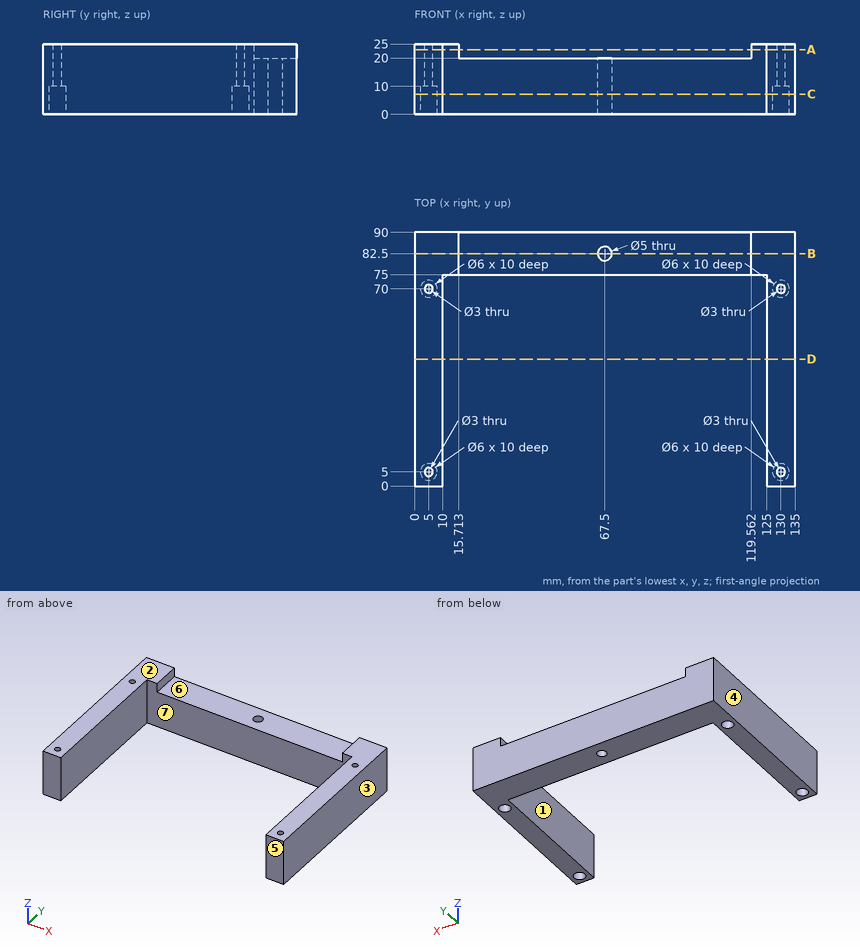
Could you check a few things on this drawing? It's one solid part, dimensions in mm from its lowest x, y, z. A direction names the side the tool comes from. Give positions to 0.01 mm unless a question says otherwise; leave off trailing zeros. Loops run counter-clockwise (first coordinate to the right, second up) from the corner with the lowest first, then second, coordinate; pieces in that order, holes last. Notation, with made-up numbers: (23, -2) -> (49, -2) arc R27 ccw to (49, 18) -> close; hole circle Ø3 at (74, 71). An arc over 180 degrees is marked (long way). Answer as CSV lines item,"result". Start each with the question number.
(1) If we section it at A-A on z = 23: Write out the boundary of the cut face in (x, y).
(2) If we section it at C-C on z = 7.25: Write out the boundary of the cut face in (x, y), then the cut area to 3 significant figures.
(3) I'm going to push flat-ended pins straight in: pin 1 Ø2 at (x, z) = (57, 17.5) entering from -Y; pin 2 Ø4.5 at (x, y) = (75, 84) entering from +Z; pin 3 Ø3 at (x, y) = (5.5, 5.5) entering from -Z. Where does each tip first touch, or does it pass through?
(4) We'd pull the mould along X, two halves only. Please class the marked faces 1, 2, 3 and 4: released by +X, released by -X, zero draft, split by the parting line, or undercut.
(5) If we section it at B-B on y = 82.5: Write out the boundary of the cut face in (x, z).
(6) I need wall thicknesses on probe 1 along X at (y, z) = (70, 15.75); probe 2 along X at (y, z) = (56, 10); probe 3 along Y at (x, z) = (129.5, 20.25) (1 decimal). Which ranges of each line are inside material? Lowest first, please.
(7) If we section it at D-D on y = 45: Write out the boundary of the cut face in (x, z), then the cut area to 3 significant figures.
(8) Which directions (+Z, -Z, +X, -X, +Y, -Y) give clear straight access to the entire face, cutting with the end or side of a thin tool? Please do the marked faces 5, 6 and 7.
Computed:
1,outline,"(0, 0) -> (10, 0) -> (10, 75) -> (15.71, 75) -> (15.71, 90) -> (0, 90) -> close; (119.56, 75) -> (125, 75) -> (125, 0) -> (135, 0) -> (135, 90) -> (119.56, 90) -> close; hole circle Ø3 at (5, 5); hole circle Ø3 at (5, 70); hole circle Ø3 at (130, 5); hole circle Ø3 at (130, 70)"
2,outline,"(0, 0) -> (10, 0) -> (10, 75) -> (125, 75) -> (125, 0) -> (135, 0) -> (135, 90) -> (0, 90) -> close; hole circle Ø6 at (5, 5); hole circle Ø6 at (5, 70); hole circle Ø5 at (67.5, 82.5); hole circle Ø6 at (130, 5); hole circle Ø6 at (130, 70)"
2,area,"3,390 mm2"
3,pin 1,"stops at y = 75"
3,pin 2,"stops at z = 20"
3,pin 3,"stops at z = 10"
4,face 1,"undercut"
4,face 2,"zero draft"
4,face 3,"released by +X"
4,face 4,"released by -X"
5,outline,"(0, 0) -> (65, 0) -> (65, 20) -> (15.71, 20) -> (15.71, 25) -> (0, 25) -> close; (70, 0) -> (135, 0) -> (135, 25) -> (119.56, 25) -> (119.56, 20) -> (70, 20) -> close"
6,probe 1,"x = 0 to 3.5, 6.5 to 10, 125 to 128.5, 131.5 to 135"
6,probe 2,"x = 0 to 10, 125 to 135"
6,probe 3,"y = 0 to 3.6, 6.4 to 68.6, 71.4 to 90"
7,outline,"(0, 0) -> (10, 0) -> (10, 25) -> (0, 25) -> close; (125, 0) -> (135, 0) -> (135, 25) -> (125, 25) -> close"
7,area,"500 mm2"
8,face 5,"+Z, -Z, +X, -X, -Y"
8,face 6,"+Z, +Y, -Y"
8,face 7,"+Z, -Z, -Y"
